```python
from build123d import *


with BuildPart() as part:
    # Szkic1 → Obrót1 (revolve)
    with BuildSketch(Plane.XY, mode=Mode.PRIVATE) as obr_t1_sk:
        Polygon((-17.5, 59.995363569), (-20, 59.995363569), (-21, 58.995363569), (-21, 51.5), (-20.5, 51.5), (-20.5, 50.995363569), (-23.5, 50.995363569), (-23.5, 44.995363569), (-20.5, 44.995363569), (-20.5, 44.5), (-21, 44.5), (-21, 8.995363569), (-20.5, 8.995363569), (-20.5, 6.495363569), (-20, 5.995363569), (-16, 5.995363569), (-16, 41.995363569), (-16.5, 42.495363569), (-16.5, 58.995363569), align=None)
    revolve(obr_t1_sk.sketch.rotate(Axis((0, 0, 0), (0, 1, 0)), 270), axis=Axis((0, 0, 0), (0, 1, 0)))


solid = part.part
```
Here's how the part is built. I have some questions about the finished solid (model axes, mm). A direction names the side the tool comes from. Round coordinates to 2 decimals unless told otherwise and drop trailing zeros. Order: outer loops, then holes, each group sorted by start corner. A loop starts at its lowest first (then second) coordinate and runs counter-clockwise, first axis right, second up. Notation, with made-up numbers: M 54.25,11 L 94.25,11 A33 ccw 94.25,48 Z; hole C 68.25,-31 d3. An arc over 180 degrees is marked long. Answer in a Markdown table with one row per item.
Item 1: Thinking about a two-plate mould opening in Y: for faces 1 (the face through (18.6, 44.5, 9.2)), 2 (the face through (18, 59.995, 0)), 3 (the face through (20.013, 7.728, 4.444)), which applies, +Y half, -Y half, draft (parallel to the pull), parting line (faces both ways), or undercut?
A:
| item | result |
|---|---|
| face 1 | undercut |
| face 2 | +Y half |
| face 3 | draft |
Item 2: For faces 4 (the face through (16.108, 50.861, 3.577)), 5 (the face through (20.013, 51.244, 4.444)), 6 (the face through (-6.31, 26.5, -20.03)), 7 (the face through (15.62, 24.25, 3.47)), which set-ups out of +Z, -Z, +X, -X, +Y, -Y let a thin tool reach every point of the face, with its end or its side?
A:
| item | result |
|---|---|
| face 4 | +Y |
| face 5 | none |
| face 6 | -Y |
| face 7 | +Y, -Y |
Item 3: Imagine slicing it at A-A, the plane y = 19.5. Write out the boundary of the cut face in (x, z), and give its area (3 significant figures).
A:
| item | result |
|---|---|
| outline | C 0,0 d42; hole C 0,0 d32 |
| area | 581 mm2 |
Item 4: I'm going to push flat-ended pins straight in: pin 1 (12.5 mm diameter, centred on x = 1.5, z = 3.5, fed in from -Y); pin 2 (5 mm diameter, centred on y = 46, z = -15, fed in from +X); pin 3 (3 mm diameter, centred on y = 17, z = 9.5, fed in from -X); pin 4 (1 mm diameter, centred on y = 43.5, z = 11, fed in from +X). Where does each tip first touch, or does it pass through?
A:
| item | result |
|---|---|
| pin 1 | passes through |
| pin 2 | stops at x = 19.9 |
| pin 3 | stops at x = -19.42 |
| pin 4 | stops at x = 18.19 |
Item 5: If I drill on L1, parallel to X at y = 20, z = 0; L2, parallel to X at y = 55, z = 0; L3, parallel to Z at x = 2, y = 34.5, over which ranges is the centre line in solid material (lowest first)? Write a range as from..to.
A:
| item | result |
|---|---|
| L1 | x = -21..-16, 16..21 |
| L2 | x = -21..-16.5, 16.5..21 |
| L3 | z = -20.9..-15.87, 15.87..20.9 |
